```python
from build123d import *

# Parameters (mm, degrees)
SKETCH3_R          = 0.8
CUT_EXTRUDE1_DEPTH = 5


with BuildPart() as part:
    # Sketch2 → Revolve1 (revolve)
    with BuildSketch(Plane.XY, mode=Mode.PRIVATE) as revolve1_sk:
        Polygon((6.1, 0), (8.1, 0), (8.1, 24), (9.95, 24), (9.95, 27), (6.1, 27), align=None)
    revolve(revolve1_sk.sketch.rotate(Axis((0, 0, 0), (0, 1, 0)), 90), axis=Axis((0, 0, 0), (0, 1, 0)))

    # Sketch3 → Cut-Extrude1 (cut)
    with BuildSketch(Plane(origin=(0, 27, 0), x_dir=(1, 0, 0), z_dir=(0, 1, 0))):
        with Locations(Location((7.72740661, -2.070552361, 0), (0, 0, 270))):
            Circle(SKETCH3_R)
        with Locations(Location((-5.656854249, -5.656854249, 0), (0, 0, 270))):
            Circle(SKETCH3_R)
        with Locations(Location((-2.070552361, 7.72740661, 0), (0, 0, 270))):
            Circle(SKETCH3_R)
        with BuildLine():
            Line((6.344154509, 2.958327832), (9.06307787, 4.226182617))
            ThreePointArc((9.06307787, 4.226182617), (9.659258263, 2.588190451), (9.961946981, 0.871557427))
            Line((9.961946981, 0.871557427), (6.973362887, 0.610090199))
            ThreePointArc((6.973362887, 0.610090199), (6.761480784, 1.811733316), (6.344154509, 2.958327832))
        make_face()
    extrude(amount=-CUT_EXTRUDE1_DEPTH, mode=Mode.SUBTRACT)


solid = part.part
```
Read the model definition and answer for the solid it produces. Units are mm, in the model's axes. A direction names the side the tool comes from. Give positions to 0.01 mm unless a question says otherwise; leave off trailing zeros. Order: outer loops, then holes, each group sorted by start corner. A loop starts at its lowest first (then second) coordinate and runs counter-clockwise, first axis right, second up.
(1) For faces 1 (the cylindrical face through (-9.71, 25.52, 2.17)), 2 (the flat face through (-8.2, 24, 1.4)), 3 (the cylindrical face through (-5.116, 25.091, 5.067)), 4 (the flat face through (7.365, 25.091, -3.434)), determine the directions among +Z, -Z, +X, -X, +Y, -Y from which every point of the face is accessible in a straight line to the end or side of a thin tool.
(2) Find section B-B (z = 0). Give the vertices of the cut face in (x, y), plus the area to 3 significant figures.
(3) Find section A-A (x = 0). Give the vertices of the cut face in (y, z).
(4) Find section C-C (y = 4). Give the vertices of the cut face in (x, z), plus the area to 3 significant figures.
(5) For a pull along X with two mould halves and no side action, classify faces 5 (the flat face through (-6, 0, 2)), 6 (the cylindrical face through (-1.83, 25.091, -6.964)), 7 (the cylindrical face through (7.907, 12.168, 1.756)) as released by +X, released by -X, zero draft, split by the parting line, or undercut.
(6) Given pin 1 (2 mm diameter, centred on x = -1.5, y = 6, fed in from +Z); pin 2 (10 mm diameter, centred on y = 3, z = -0.5, fed in from +X); pin 3 (5 mm diameter, centred on y = 23.5, z = 3.5, fed in from +X), each flat-ended and moving along its own axis, determine where each tip first touches the part or whether it passes through.
(7) Straight lines are drawn through the part: L1, parallel to X at y = 25, z = 5; L2, parallel to X at y = 4.75, z = 0; L3, parallel to Y at x = 7, z = 7. For each, find the intervals that lie inside material, in ascending order.
(8) Find section D-D (x = -7). Give the vertices of the cut face in (y, z).
Result sheet:
1. face 1: +Y, -Y
1. face 2: -Y
1. face 3: +Y
1. face 4: +X, +Y
2. outline: (-9.95, 24) - (-8.1, 24) - (-8.1, 0) - (-6.1, 0) - (-6.1, 27) - (-9.95, 27) - close; (6.1, 0) - (8.1, 0) - (8.1, 24) - (9.95, 24) - (9.95, 27) - (6.1, 27) - close
2. area: 119 mm2
3. outline: (0, -8.1) - (24, -8.1) - (24, -9.95) - (27, -9.95) - (27, -6.1) - (0, -6.1) - close; (0, 6.1) - (27, 6.1) - (27, 9.95) - (24, 9.95) - (24, 8.1) - (0, 8.1) - close
4. outline: circle Ø16.2 at (0, 0); hole circle Ø12.2 at (0, 0)
4. area: 89.2 mm2
5. face 5: zero draft
5. face 6: undercut
5. face 7: split by the parting line
6. pin 1: stops at z = 8.08
6. pin 2: stops at x = 8.1
6. pin 3: stops at x = 9.89
7. L1: x = -8.6 to -6.11, -5.2 to -3.49, 3.49 to 8.6
7. L2: x = -8.1 to -6.1, 6.1 to 8.1
7. L3: y = 24 to 27
8. outline: (0, -4.08) - (24, -4.08) - (24, -7.07) - (27, -7.07) - (27, 7.07) - (24, 7.07) - (24, 4.08) - (0, 4.08) - close
